Read the model definition and answer for the solid it produces. Units are mm, in the model's axes. A direction names the side the tool comes from. Round coordinates to 2 decimals unless told otherwise and drop trailing zeros. Write each loop counter-clockwise with the first axis right and the second up, starting at its lowest first coordinate (ties: lowest second). Pieces come first, ordered by that corner, then holes. Notation, with made-up numbers: (-35, -7) - (-12, -7) arc R15 cw to (-12, 12) - close; hole circle Ø10 at (19, -39.75). An arc over 180 degrees is marked (long way). Use one line per item in the form item = value. Start each with the question number.
1) Each of these flat-tipped pins is pushed along its axis until it touches: pin 1 (8 mm diameter, centred on x = -9.5, y = -10, fed in from -Z); pin 2 (2.5 mm diameter, centred on y = 28.5, z = -10.5, fed in from +X); pin 3 (11 mm diameter, centred on y = 33.5, z = -7, fed in from -X). Where does it stop, or does it pass through?
2) The part is cut by section A-A, the plane y = 0. Give the vertices of the cut face in (x, z), plus the area to 3 significant figures.
3) For faces 1 (the face through (3.6, 28, -10)), 2 (the face through (-1, 18, 0.8)), 3 (the face through (1.775, 35.028, -12.832)), 4 (the face through (-20, 6, 1)), determine the directions among +Z, -Z, +X, -X, +Y, -Y from which every point of the face is accessible in a straight line to the end or side of a thin tool.
4) The part is cut by section C-C, the plane z = -9.7. Give the vertices of the cut face in (x, y), plus the area to 3 significant figures.
5) Consider line 1 along Y through (x, z) = (8, 0.6); line 2 along X through (y, z) = (-20, 1.35); line 3 along Y through (x, z) = (0, 1.3). Determine where each line is inside the solid, lowest interval first. Write a range as from..to.
6) The part is cut by section B-B, the plane x = 8. Give the vertices of the cut face in (y, z), plus the area to 3 significant figures.
7) The part is cut by section D-D, the plane y = -20. Give the vertices of the cut face in (x, z), plus the area to 3 significant figures.
8) For a pull along Y with two mould halves and no side action, classify faces 5 (the face through (-19.4, 36.43, 1.52)), 6 (the face through (1, -18, 0.8)), 7 (the face through (6.1, 32.07, -16.14)) as released by +Y, released by -Y, zero draft, split by the parting line, or undercut.
from build123d import *

# Parameters (mm, degrees)
SKETCH_1_W          = 40
SKETCH_1_H          = 62
SKETCH_1_R          = 2
SKETCH_1_R_2        = 2.7
EXTRUDE_1_DEPTH     = 3
SKETCH_3_W          = 14
SKETCH_3_H          = 10
EXTRUDE_2_DEPTH     = 17
CUT_EXTRUDE_START   = -10
CUT_EXTRUDE_1_DEPTH = 4
CUT_EXTRUDE_2_REACH = 65.663
SKETCH_6_R          = 2.2
FILLET_1_R          = 3
CHAMFER_1_SIZE      = 4
CUT_EXTRUDE_3_DEPTH = 3
FILLET_2_R          = 2
SKETCH_7_R          = 5
SKETCH_7_R_2        = 3
CUT_EXTRUDE_4_DEPTH = 0.8


with BuildPart() as part:
    # 草图1 → 凸台-拉伸1 (new body)
    with BuildSketch(Plane.XY):
        with Locations((0, 6)):
            Rectangle(SKETCH_1_W, SKETCH_1_H)
        with Locations((0, 20)):
            Circle(SKETCH_1_R, mode=Mode.SUBTRACT)
        with Locations((8, 20)):
            Circle(SKETCH_1_R, mode=Mode.SUBTRACT)
        with Locations((-8, -20)):
            Circle(SKETCH_1_R, mode=Mode.SUBTRACT)
        with Locations((0, -20)):
            Circle(SKETCH_1_R, mode=Mode.SUBTRACT)
        with Locations((8, -20)):
            Circle(SKETCH_1_R, mode=Mode.SUBTRACT)
        with Locations((-8, 20)):
            Circle(SKETCH_1_R, mode=Mode.SUBTRACT)
        Circle(SKETCH_1_R_2, mode=Mode.SUBTRACT)
    extrude(amount=EXTRUDE_1_DEPTH)

    # 草图3 → 凸台-拉伸2 (add)
    with BuildSketch(Plane(origin=(0, 0, 0), x_dir=(-1, 0, 0), z_dir=(0, 0, -1))):
        with Locations((0, 32)):
            Rectangle(SKETCH_3_W, SKETCH_3_H)
    extrude(amount=EXTRUDE_2_DEPTH)

    # 草图5 → 切除-拉伸1 (cut)
    with BuildSketch(Plane.XZ.offset(-27).offset(CUT_EXTRUDE_START)):
        Polygon((3.6, -11.778460969), (3.6, -7.621539031), (0, -5.543078062), (-3.6, -7.621539031), (-3.6, -11.778460969), (0, -13.856921938), align=None)
    extrude(amount=CUT_EXTRUDE_1_DEPTH, mode=Mode.SUBTRACT)

    # 草图6 → 切除-拉伸2 (cut, up to next)
    with BuildSketch(Plane(origin=(0, 33, 0), x_dir=(-1, 0, 0), z_dir=(0, 1, 0)), mode=Mode.PRIVATE) as cut_extrude_2_sk1:
        with Locations(Location((0, -9.7, 0), (0, 0, 90))):
            Circle(SKETCH_6_R)
    cut_extrude_2_tool1 = extrude(cut_extrude_2_sk1.sketch, amount=-CUT_EXTRUDE_2_REACH, mode=Mode.PRIVATE) & part.part
    add(cut_extrude_2_tool1.solids().sort_by_distance((0, 33, -9.7))[0], mode=Mode.SUBTRACT)

    # 圆角1
    fillet_1_edges = [part.edges().sort_by_distance(p)[0] for p in [
        (-7, 32, -17),
        (7, 32, -17),
    ]]
    fillet(fillet_1_edges, radius=FILLET_1_R)

    # 倒角1
    chamfer_1_edges = [part.edges().sort_by_distance(p)[0] for p in [
        (-7, 32, 0),
        (7, 32, 0),
    ]]
    chamfer(chamfer_1_edges, length=CHAMFER_1_SIZE)

    # 草图5<2> → 切除-拉伸3 (cut)
    with BuildSketch(Plane.XZ.offset(-27)):
        Polygon((3.6, -11.778460969), (3.6, -7.621539031), (0, -5.543078062), (-3.6, -7.621539031), (-3.6, -11.778460969), (0, -13.856921938), align=None)
    extrude(amount=-CUT_EXTRUDE_3_DEPTH, mode=Mode.SUBTRACT)

    # 圆角2
    fillet_2_edges = [part.edges().sort_by_distance(p)[0] for p in [
        (-20, 37, 1.5),
        (20, 37, 1.5),
        (20, -25, 1.5),
        (-20, -25, 1.5),
    ]]
    fillet(fillet_2_edges, radius=FILLET_2_R)

    # 草图7 → 切除-拉伸4 (cut)
    with BuildSketch(Plane(origin=(0, 0, 0), x_dir=(-1, 0, 0), z_dir=(0, 0, -1))):
        Circle(SKETCH_7_R)
        with Locations((-8, 20)):
            Circle(SKETCH_7_R_2)
        with Locations((0, 20)):
            Circle(SKETCH_7_R_2)
        with Locations(Location((8, 20, 0), (0, 0, 180))):
            Circle(SKETCH_7_R_2)
        with Locations((8, -20)):
            Circle(SKETCH_7_R_2)
        with Locations(Location((0, -20, 0), (0, 0, 180))):
            Circle(SKETCH_7_R_2)
        with Locations(Location((-8, -20, 0), (0, 0, 180))):
            Circle(SKETCH_7_R_2)
    extrude(amount=-CUT_EXTRUDE_4_DEPTH, mode=Mode.SUBTRACT)


solid = part.part
Geometry results:
q1.pin_1 = 0
q1.pin_2 = 7
q1.pin_3 = -9.5
q2.outline = (-20, 0) - (-5, 0) - (-5, 0.8) - (-2.7, 0.8) - (-2.7, 3) - (-20, 3) - close; (2.7, 0.8) - (5, 0.8) - (5, 0) - (20, 0) - (20, 3) - (2.7, 3) - close
q2.area = 100 mm2
q3.face_1 = -Y
q3.face_2 = -Z
q3.face_3 = +Y
q3.face_4 = +Z, -Z, -X, +Y, -Y
q4.outline = (-7, 27) - (-3.6, 27) - (-3.6, 30) - (-2.2, 30) - (-2.2, 33) - (-3.6, 33) - (-3.6, 37) - (-7, 37) - close; (2.2, 30) - (3.6, 30) - (3.6, 27) - (7, 27) - (7, 37) - (3.6, 37) - (3.6, 33) - (2.2, 33) - close
q4.area = 76.4 mm2
q5.line_1 = -25..-23, -17..17, 23..37
q5.line_2 = -20..-10, -6..-2, 2..6, 10..20
q5.line_3 = -25..-22, -18..-2.7, 2.7..18, 22..37
q6.outline = (-25, 0) - (-23, 0) - (-23, 0.8) - (-22, 0.8) - (-22, 3) - (-25, 3) - close; (-18, 0.8) - (-17, 0.8) - (-17, 0) - (17, 0) - (17, 0.8) - (18, 0.8) - (18, 3) - (-18, 3) - close; (22, 0.8) - (23, 0.8) - (23, 0) - (27, 0) - (27, -3) - (37, -3) - (37, 3) - (22, 3) - close
q6.area = 189 mm2
q7.outline = (-20, 0) - (-11, 0) - (-11, 0.8) - (-10, 0.8) - (-10, 3) - (-20, 3) - close; (-6, 0.8) - (-5, 0.8) - (-5, 0) - (-3, 0) - (-3, 0.8) - (-2, 0.8) - (-2, 3) - (-6, 3) - close; (2, 0.8) - (3, 0.8) - (3, 0) - (5, 0) - (5, 0.8) - (6, 0.8) - (6, 3) - (2, 3) - close; (10, 0.8) - (11, 0.8) - (11, 0) - (20, 0) - (20, 3) - (10, 3) - close
q7.area = 79.2 mm2
q8.face_5 = released by +Y
q8.face_6 = undercut
q8.face_7 = zero draft
